Can you work these out from the model? Positions are in its coordinate system, mm. A direction names the side the tool comes from. Give positions to 0.01 mm unless a question says otherwise; leave off trailing zeros. Write each loop counter-clockwise with the first axis right and the second up, starting at its lowest first coordinate (ties: lowest second). Pieces come first, ordered by that corner, then holes. Notation, with made-up numbers: (8, -1.5) - (27, -1.5) arc R20 ccw to (27, 27.5) - close; hole circle Ø2 at (48, -20.75). An arc over 180 degrees is marked (long way). Return JSON: item names as keys, results as strings. Group by question number.
from build123d import *

# Parameters (mm, degrees)
SKETCH2_W = 2
SKETCH2_H = 1.5
FILLET1_R = 1
FILLET2_R = 1


with BuildPart() as part:
    # Sketch1 → Revolve1 (revolve)
    with BuildSketch(Plane.XY, mode=Mode.PRIVATE) as revolve1_sk:
        Polygon((0, 0), (10, 0), (10, 0.5), (8, 0.5), (7.521875, 1), (2.522875817, 1), (2, 0.5), (0, 0.5), align=None)
    revolve(revolve1_sk.sketch.rotate(Axis((-1.430896147, -1, 0), (1, 0, 0)), 90), axis=Axis((-1.430896147, -1, 0), (1, 0, 0)))

    # Sketch2 → Revolve2 (revolve)
    with BuildSketch(Plane.XY, mode=Mode.PRIVATE) as revolve2_sk:
        with Locations((11, -2.75)):
            Rectangle(SKETCH2_W, SKETCH2_H)
    revolve(revolve2_sk.sketch.rotate(Axis((10, -1, 0), (1, 0, 0)), 270), axis=Axis((10, -1, 0), (1, 0, 0)))

    # Fillet1
    fillet1_edges = [part.edges().sort_by_distance(p)[0] for p in [
        (2.522875817, -1, -2),
        (7.521875, -1, -2),
    ]]
    fillet(fillet1_edges, radius=FILLET1_R)

    # Fillet2
    fillet2_edges = [part.edges().sort_by_distance(p)[0] for p in [
        (12, -1, -2.5),
        (10, -1, -2.5),
    ]]
    fillet(fillet2_edges, radius=FILLET2_R - 0.0001)  # a hair under: the kernel refuses the full size


solid = part.part
1) I need wall thicknesses on line 1 along Y through (x, z) = (8.25, 0); line 2 along Z through (x, y) = (7.25, -2.3); line 3 along Z through (x, y) = (11, -0.45). Which ranges of each line are inside material? Lowest first, please.
2) Imagine slicing it at A-A, the plane x = 5.75. Write out the boundary of the cut face in (y, z).
3) On a 3-axis mill with a long thin cutter (end or side, diameter ignored), from which of +Z, -Z, +X, -X, +Y, -Y can I reach the whole of each face in a straight line? I mean faces 3 (the face through (8.99, -1.45, 1.43)), 4 (the face through (0.99, -1.45, 1.43)). Say none if no direction works.
4) Will these pins go through, and if not, where does the flat tip stop? pin 1 Ø3 at (x, z) = (9, -0.5) entering from -Y; pin 2 Ø2 at (x, y) = (5, -2) entering from -Z; pin 3 Ø3 at (x, z) = (2.5, -1) entering from +Y.
5) We'd pull the mould along Y, two halves only. Please class faces 1 (the face through (4.98, -1.601, 1.908)), 2 (the face through (6, 0, 0)): pulls with the +Y half, pulls with the -Y half, needs draft (parallel to the pull), parting line crosses it, or undercut.
6) Imagine slicing it at B-B, the plane x = 9.75. Write out the boundary of the cut face in (y, z), and give its area (3 significant figures).
Resolved:
{
 "1": {"line 1": "-2.5 to -2, 0 to 0.5", "line 2": "-1.5 to 1.5", "line 3": "-2.44 to -0.84, 0.84 to 2.44"},
 "2": {"outline": "circle Ø4 at (-1, 0); hole circle Ø2 at (-1, 0)"},
 "3": {"face 3": "none", "face 4": "-X"},
 "4": {"pin 1": "y = -3.34", "pin 2": "z = -2", "pin 3": "y = 1"},
 "5": {"face 1": "parting line crosses it", "face 2": "undercut"},
 "6": {"outline": "circle Ø3 at (-1, 0); hole circle Ø2 at (-1, 0)", "area": "3.93 mm^2"}
}
